Read the model definition and answer for the solid it produces. Units are mm, in the model's axes. A direction names the side the tool comes from. Coordinates: 2 decimals unless noted, no trailing zeros. Loops run counter-clockwise (first coordinate to the right, second up) from the corner with the lowest first, then second, coordinate; pieces in that order, holes last. Notation, with made-up numbers: M 64,47.25 L 106,47.25 A23 cw 106,60.25 Z; hole C 13.5,49.5 d3. An arc over 180 degrees is marked long. One line per item, written item: value. Start each with the question number.
1. Flat-ended cylindrical pins translate along their axes: pin 1 (3 mm diameter, centred on x = 5, z = 1, fed in from -Y); pin 2 (1.5 mm diameter, centred on y = -5.5, z = -4.5, fed in from +X); pin 3 (1 mm diameter, centred on y = -4.5, z = 1.5, fed in from +X); pin 4 (3 mm diameter, centred on y = -29, z = 0.5, fed in from -X). Find the tip coordinate at first contact, or state that the pin passes through.
2. For faces 1 (the face through (0, 0, 5)), 2 (the face through (-3.61, 5.32, 6.21)), determine the directions among +Z, -Z, +X, -X, +Y, -Y from which every point of the face is accessible in a straight line to the end or side of a thin tool.
3. The part is cut by section A-A (y = -28.5). Write down the section's boundary in (x, z), then the cut area to 3 significant figures.
4. Consider probe 1 along Y at (x, z) = (-1.75, -5.5); probe 2 along Z at (x, y) = (-3.5, -19.5); probe 3 along Z at (x, y) = (1.5, -2). Determine where each line is inside the solid, lowest interval first.
```python
from build123d import *

# Parameters (mm, degrees)
SKETCH_2_OUTSIDE_W  = 26.932
SKETCH_2_OUTSIDE_H  = 26.932
CUT_EXTRUDE_1_DEPTH = 5.5
CUT_EXTRUDE_START   = 5.5
SKETCH_3_OUTSIDE_W  = 34.642
SKETCH_3_OUTSIDE_H  = 32.498
SKETCH_3_OUTSIDE_R  = 6.92820323
CUT_EXTRUDE_2_DEPTH = 2.75
CUT_EXTRUDE_2_DRAFT = -55
CHAMFER_1_SIZE      = 0.3


with BuildPart() as part:
    # 草图1 → 旋转1 (revolve)
    with BuildSketch(Plane.XY, mode=Mode.PRIVATE) as revolve_1_sk:
        Polygon((0, 5.5), (8, 5.5), (8, 0), (4.545454545, 0), (4.545454545, -33), (0, -33), align=None)
    revolve(revolve_1_sk.sketch.rotate(Axis((0, 0, 0), (0, 1, 0)), 90), axis=Axis((0, 0, 0), (0, 1, 0)))

    # 草图2 outside → 切除-拉伸1 (cut)
    with BuildSketch(Plane(origin=(0, 0, 0), x_dir=(1, 0, 0), z_dir=(0, 1, 0))):
        Rectangle(SKETCH_2_OUTSIDE_W, SKETCH_2_OUTSIDE_H)
        Polygon((8, 0), (4, 6.92820323), (-4, 6.92820323), (-8, 0), (-4, -6.92820323), (4, -6.92820323), align=None, mode=Mode.SUBTRACT)
    extrude(amount=CUT_EXTRUDE_1_DEPTH, mode=Mode.SUBTRACT)


with BuildPart() as cut_extrude_2_tool:
    # 草图3 outside → 切除-拉伸2 (with draft: the straight prism first)
    with BuildSketch(Plane(origin=(0, 0, 0), x_dir=(1, 0, 0), z_dir=(0, 1, 0)).offset(CUT_EXTRUDE_START)):
        Rectangle(SKETCH_3_OUTSIDE_W, SKETCH_3_OUTSIDE_H)
        Circle(SKETCH_3_OUTSIDE_R, mode=Mode.SUBTRACT)
    extrude(amount=-CUT_EXTRUDE_2_DEPTH)
    # 切除-拉伸2: the draft: its side faces are tilted about the plane it starts from
    cut_extrude_2_sides = [cut_extrude_2_tool.faces().sort_by_distance(p)[0] for p in [
        (0, 4.125, 16.249),
        (17.321, 4.125, 0),
        (0, 4.125, -16.249),
        (-17.321, 4.125, 0),
        (-6.92820323, 4.125, 0),
    ]]
    draft(cut_extrude_2_sides, Plane(origin=(0, 0, 0), x_dir=(1, 0, 0), z_dir=(0, 1, 0)).offset(CUT_EXTRUDE_START), CUT_EXTRUDE_2_DRAFT)


with BuildPart() as part_1:
    add(part.part)

    # 切除-拉伸2: cut by cut_extrude_2_tool
    add(cut_extrude_2_tool.part, mode=Mode.SUBTRACT)

    # 倒角1
    chamfer_1_edges = [part_1.edges().sort_by_distance(p)[0] for p in [
        (0, -33, 4.545454545),
    ]]
    chamfer(chamfer_1_edges, length=CHAMFER_1_SIZE)


solid = part_1.part
```
Answer block:
1. pin 1: stops at y = -33
1. pin 2: stops at x = 2.57
1. pin 3: stops at x = 4.43
1. pin 4: stops at x = -4.55
2. face 1: -Y
2. face 2: +Z, -X, +Y
3. outline: C 0,0 d9.09
3. area: 64.9 mm2
4. probe 1: y = 0 to 5.5
4. probe 2: z = -2.9 to 2.9
4. probe 3: z = -4.29 to 4.29
